CAD build for the part. Positions are in the model's coordinates, mm. Round coordinates to 2 decimals unless told otherwise and drop trailing zeros. Write each loop counter-clockwise with the first axis right and the second up, starting at its lowest first coordinate (ties: lowest second). Pieces come first, ordered by that corner, then holes. Notation, with made-up numbers: (-24, -39.5) -> (-19, -39.5) arc R11 ccw to (-19, -35.5) -> close; hole circle Ø9 at (37.5, 63.25). An arc over 180 degrees is marked (long way). Answer in a Markdown table with one row per item. Add a question column.
```python
from build123d import *

# Parameters (mm, degrees)
F0_W     = 75
F0_H     = 36
F1_DEPTH = 36
F2_R     = 2


with BuildPart() as f1:
    # F0 (on Top) → F1 (new body)
    with BuildSketch(Plane.XY):
        Rectangle(F0_W, F0_H)
        Polygon((-8.825392, 7.5), (-8.825392, 8), (-8.825392, 8.5), (8.995996, 8.5), (8.995996, 8), (8.995996, 7.5), align=None, mode=Mode.SUBTRACT)
    extrude(amount=F1_DEPTH)

    # F2
    f2_edges = [f1.edges().sort_by_distance(p)[0] for p in [
        (0, -18, 36),
        (37.5, -18, 18),
        (37.5, 0, 36),
        (37.5, 18, 18),
        (37.5, 0, 0),
        (0, -18, 0),
        (-37.5, -18, 18),
        (0, 18, 0),
        (-37.5, 0, 0),
        (-37.5, 18, 18),
        (-37.5, 0, 36),
        (0, 18, 36),
    ]]
    fillet(f2_edges, radius=F2_R)


solid = f1.part
```
Item 1: Saw through at A-A on x = 0. Give the cut face in (y, z), then the cut area to 3 significant figures.
Item 2: Drill centre lines: probe 1 along Y at (x, z) = (0.5, 28); probe 2 along X at (y, z) = (8, 20). Where is each one in solid material? Low to high.
Item 3: Two-plate mould, pull along Y, no slides. Class faces 1 (the flat face through (0, 8.5, 18)), 2 (the flat face through (0, 7.5, 18)), 3 (the cylindrical face through (36.93, 0.22, 0.6)), 4 (the flat face through (0, -18, 18)): +Y half, -Y half, draft (parallel to the pull), parting line (faces both ways), or undercut.
Recorded:
| question | item | result |
|---|---|---|
| 1 | outline | (-18, 2) arc R2 ccw to (-16, 0) -> (7.5, 0) -> (7.5, 36) -> (-16, 36) arc R2 ccw to (-18, 34) -> close; (8.5, 0) -> (16, 0) arc R2 ccw to (18, 2) -> (18, 34) arc R2 ccw to (16, 36) -> (8.5, 36) -> close |
| 1 | area | 1,260 mm2 |
| 2 | probe 1 | -18 to 7.5, 8.5 to 18 |
| 2 | probe 2 | -37.5 to -8.83, 9 to 37.5 |
| 3 | face 1 | undercut |
| 3 | face 2 | undercut |
| 3 | face 3 | draft |
| 3 | face 4 | -Y half |
